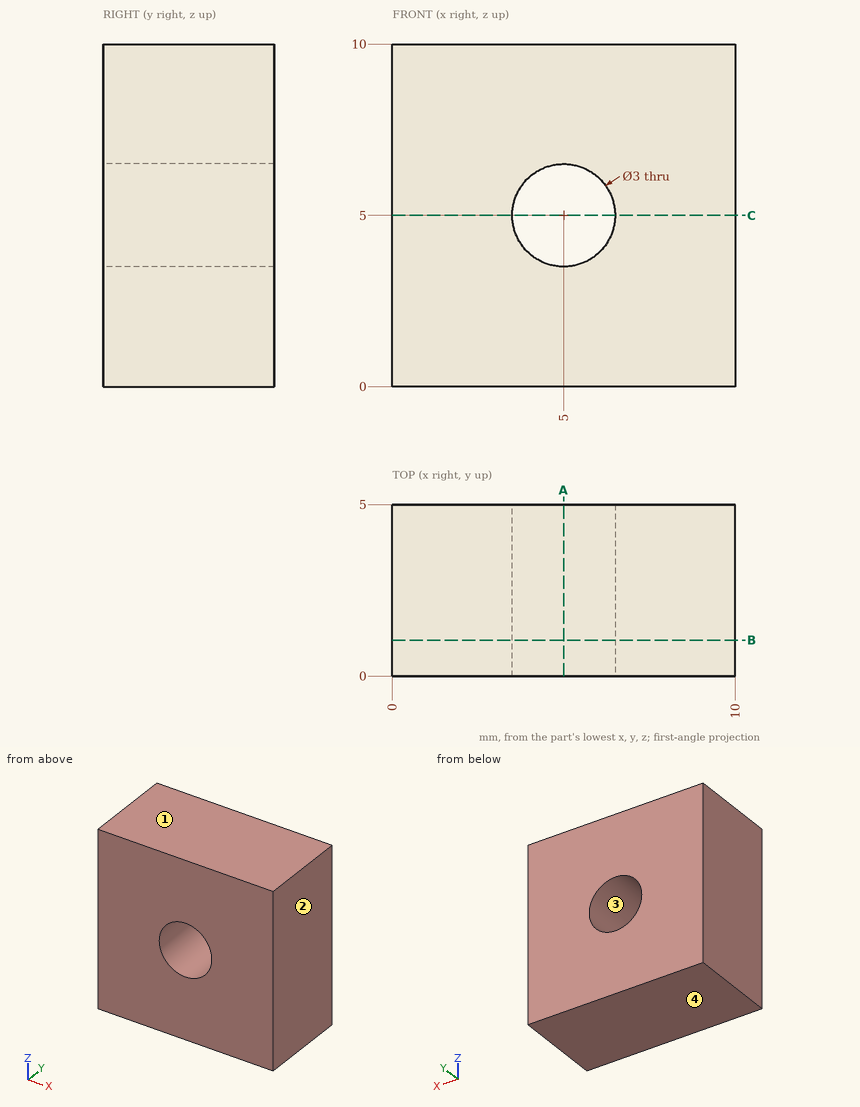
Check sheet for the drawn part. Datum: minimum x, y, z corner. Units: mm. Coordinates: 2 decimals unless noted, no trailing zeros. Loops run counter-clockwise (first coordinate to the right, second up) from the corner with the lowest first, then second, coordinate; pieces in that order, holes last. Notation, with made-up numbers: (4, 43) -> (23, 43) arc R22 ccw to (23, 65) -> close; hole circle Ø3 at (-18.5, 84.25). An arc over 180 degrees is marked (long way). Answer as a JSON object with one key per item and string values. Group by question number.
Item 1: Sectioned sample at B-B on y = 1.05. Record the boundary of the cut face in (x, z), plus the area to 3 significant figures.
Item 2: Mould release check, pull along Z, two halves, no side actions. Record for the marked faces 1, 2, 3 and 4: +Z half, -Z half, draft (parallel to the pull), parting line (faces both ways), or undercut.
Item 3: Sectioned sample at C-C on z = 5. Record the boundary of the cut face in (x, y), plus the area to 3 significant figures.
Item 4: Sectioned sample at A-A on x = 5. Record the boundary of the cut face in (y, z), plus the area to 3 significant figures.
Item 5: Scan lines: probe 1 along Z at (x, y) = (5, 1.45); probe 2 along X at (y, z) = (4.5, 4.25); probe 3 along Z at (x, y) = (4.5, 1.5). Record each from-to range of solid material in increasing order.
Evaluation:
{
 "1": {"outline": "(0, 0) -> (10, 0) -> (10, 10) -> (0, 10) -> close; hole circle Ø3 at (5, 5)", "area": "92.9 mm²"},
 "2": {"face 1": "+Z half", "face 2": "draft", "face 3": "undercut", "face 4": "-Z half"},
 "3": {"outline": "(0, 0) -> (3.5, 0) -> (3.5, 5) -> (0, 5) -> close; (6.5, 0) -> (10, 0) -> (10, 5) -> (6.5, 5) -> close", "area": "35.0 mm²"},
 "4": {"outline": "(0, 0) -> (5, 0) -> (5, 3.5) -> (0, 3.5) -> close; (0, 6.5) -> (5, 6.5) -> (5, 10) -> (0, 10) -> close", "area": "35.0 mm²"},
 "5": {"probe 1": "z = 0 to 3.5, 6.5 to 10", "probe 2": "x = 0 to 3.7, 6.3 to 10", "probe 3": "z = 0 to 3.59, 6.41 to 10"}
}
